```python
from build123d import *

# Parameters (mm, degrees)
SKETCH1_R               = 29.75
BOSS_EXTRUDE1_DEPTH     = 40
CUT_EXTRUDE1_DEPTH      = 4
CUT_EXTRUDE1_DEPTH_BACK = 4
CUT_EXTRUDE1_START      = -20
CUT_EXTRUDE3_START      = -16
CUT_EXTRUDE3_DEPTH      = 16


with BuildPart() as part:
    # Sketch1 → Boss-Extrude1 (new body)
    with BuildSketch(Plane.XY):
        Circle(SKETCH1_R)
        with BuildLine():
            Line((1.5, 2), (1.5, 3.97649343))
            ThreePointArc((1.5, 3.97649343), (0, 4.25), (-1.5, 3.97649343))
            Line((-1.5, 3.97649343), (-1.5, 2))
            ThreePointArc((-1.5, 2), (-2.5, 0), (-1.5, -2))
            Line((-1.5, -2), (-1.5, -3.97649343))
            ThreePointArc((-1.5, -3.97649343), (0, -4.25), (1.5, -3.97649343))
            Line((1.5, -3.97649343), (1.5, -2))
            ThreePointArc((1.5, -2), (2.5, 0), (1.5, 2))
        make_face(mode=Mode.SUBTRACT)
    extrude(amount=BOSS_EXTRUDE1_DEPTH)

    # Sketch2 → Cut-Extrude1 (cut, two sides: drawn at the far end of the back side and taken through both)
    with BuildSketch(Plane.XY.offset(40).offset(CUT_EXTRUDE1_START - CUT_EXTRUDE1_DEPTH_BACK)):
        with BuildLine():
            Line((2.621054601, -11.710255026), (6.498031199, -29.031673919))
            ThreePointArc((6.498031199, -29.031673919), (3.268807192, -29.569873174), (0, -29.75))
            Line((0, -29.75), (0, -12))
            ThreePointArc((0, -12), (1.318510464, -11.927343801), (2.621054601, -11.710255026))
        make_face()
        with BuildLine():
            Line((5.202633875, -10.813537847), (12.898196481, -26.808562579))
            ThreePointArc((12.898196481, -26.808562579), (9.874487797, -28.06344581), (6.731205322, -28.978498493))
            Line((6.731205322, -28.978498493), (2.715108029, -11.688806115))
            ThreePointArc((2.715108029, -11.688806115), (3.982986674, -11.319709234), (5.202633875, -10.813537847))
        make_face()
        with BuildLine():
            Line((7.514375173, -9.355969525), (18.62938845, -23.195007781))
            ThreePointArc((18.62938845, -23.195007781), (15.968021699, -25.101489657), (13.113292322, -26.704008397))
            Line((13.113292322, -26.704008397), (5.289395222, -10.771364732))
            ThreePointArc((5.289395222, -10.771364732), (6.440882702, -10.124970618), (7.514375173, -9.355969525))
        make_face()
        with BuildLine():
            Line((9.436378538, -7.413147786), (23.394355125, -18.378428885))
            ThreePointArc((23.394355125, -18.378428885), (21.233363816, -20.837628489), (18.815249924, -23.044497614))
            Line((18.815249924, -23.044497614), (7.589344507, -9.295259542))
            ThreePointArc((7.589344507, -9.295259542), (8.564718178, -8.405093844), (9.436378538, -7.413147786))
        make_face()
        with BuildLine():
            Line((10.868958019, -5.085838336), (26.945958422, -12.608640875))
            ThreePointArc((26.945958422, -12.608640875), (25.397423769, -15.493010227), (23.541342405, -18.189769041))
            Line((23.541342405, -18.189769041), (9.495667525, -7.337049697))
            ThreePointArc((9.495667525, -7.337049697), (10.244338999, -6.249281436), (10.868958019, -5.085838336))
        make_face()
        with BuildLine():
            Line((11.737811955, -2.494748588), (29.099992138, -6.184897541))
            ThreePointArc((29.099992138, -6.184897541), (28.244229893, -9.344836957), (27.046447919, -12.391616317))
            Line((27.046447919, -12.391616317), (10.909491598, -4.998299019))
            ThreePointArc((10.909491598, -4.998299019), (11.392630545, -3.769345999), (11.737811955, -2.494748588))
        make_face()
        with BuildLine():
            Line((11.997876673, 0.225732911), (29.744735918, 0.559629508))
            ThreePointArc((29.744735918, 0.559629508), (29.626130745, -2.711987667), (29.148771898, -5.95076439))
            Line((29.148771898, -5.95076439), (11.757487825, -2.400308325))
            ThreePointArc((11.757487825, -2.400308325), (11.950035931, -1.093910992), (11.997876673, 0.225732911))
        make_face()
        with BuildLine():
            Line((11.635663748, 2.934506626), (28.846749709, 7.275131011))
            ThreePointArc((28.846749709, 7.275131011), (29.471453141, 4.061520619), (29.739275948, 0.798727786))
            Line((29.739275948, 0.798727786), (11.995674332, 0.322175914))
            ThreePointArc((11.995674332, 0.322175914), (11.887644965, 1.638260418), (11.635663748, 2.934506626))
        make_face()
        with BuildLine():
            Line((10.669959589, 5.491080255), (26.452608147, 13.613303133))
            ThreePointArc((26.452608147, 13.613303133), (27.788219537, 10.624375509), (28.787333194, 7.506793428))
            Line((28.787333194, 7.506793428), (11.611697423, 3.02795029))
            ThreePointArc((11.611697423, 3.02795029), (11.208693595, 4.28546239), (10.669959589, 5.491080255))
        make_face()
        with BuildLine():
            Line((9.150851066, 7.762855451), (22.686484935, 19.245412473))
            ThreePointArc((22.686484935, 19.245412473), (24.663731933, 16.636190283), (26.342316763, 13.825514368))
            Line((26.342316763, 13.825514368), (10.625472308, 5.576678065))
            ThreePointArc((10.625472308, 5.576678065), (9.948396074, 6.710396081), (9.150851066, 7.762855451))
        make_face()
        with BuildLine():
            Line((7.157127728, 9.632005123), (17.743712492, 23.879346034))
            ThreePointArc((17.743712492, 23.879346034), (20.260043902, 21.785158276), (22.531039016, 19.427166053))
            Line((22.531039016, 19.427166053), (9.088150191, 7.83616782))
            ThreePointArc((9.088150191, 7.83616782), (8.172118549, 8.787290733), (7.157127728, 9.632005123))
        make_face()
        with BuildLine():
            Line((4.792195325, 11.001584611), (11.880650911, 27.274761849))
            ThreePointArc((11.880650911, 27.274761849), (14.805555575, 25.804224928), (17.551174341, 24.021215191))
            Line((17.551174341, 24.021215191), (7.07946528, 9.689229657))
            ThreePointArc((7.07946528, 9.689229657), (5.971988803, 10.408426862), (4.792195325, 11.001584611))
        make_face()
        with BuildLine():
            Line((2.178712609, 11.80055979), (5.401391677, 29.25555448))
            ThreePointArc((5.401391677, 29.25555448), (8.583167521, 28.484938745), (11.661006643, 27.369388449))
            Line((11.661006643, 27.369388449), (4.703599318, 11.039753324))
            ThreePointArc((4.703599318, 11.039753324), (3.462117992, 11.489723191), (2.178712609, 11.80055979))
        make_face()
        with BuildLine():
            Line((-0.547770447, 11.987491295), (-1.358014233, 29.718988834))
            ThreePointArc((-1.358014233, 29.718988834), (1.915607925, 29.68826277), (5.166033286, 29.298030652))
            Line((5.166033286, 29.298030652), (2.083778132, 11.817693036))
            ThreePointArc((2.083778132, 11.817693036), (0.772682188, 11.975097588), (-0.547770447, 11.987491295))
        make_face()
    extrude(amount=CUT_EXTRUDE1_DEPTH + CUT_EXTRUDE1_DEPTH_BACK, mode=Mode.SUBTRACT)

    # Sketch3 → Cut-Extrude3 (cut)
    with BuildSketch(Plane.XY.offset(40).offset(CUT_EXTRUDE3_START)):
        with BuildLine():
            Line((0, -12), (0, -18))
            ThreePointArc((0, -18), (1.977765696, -17.891015702), (3.931581902, -17.565382539))
            Line((3.931581902, -17.565382539), (2.621054601, -11.710255026))
            ThreePointArc((2.621054601, -11.710255026), (1.318510464, -11.927343801), (0, -12))
        make_face()
        with BuildLine():
            Line((2.715108029, -11.688806115), (4.072662044, -17.533209172))
            ThreePointArc((4.072662044, -17.533209172), (5.974480012, -16.979563852), (7.803950812, -16.22030677))
            Line((7.803950812, -16.22030677), (5.202633875, -10.813537847))
            ThreePointArc((5.202633875, -10.813537847), (3.982986674, -11.319709234), (2.715108029, -11.688806115))
        make_face()
        with BuildLine():
            Line((5.289395222, -10.771364732), (7.934092833, -16.157047098))
            ThreePointArc((7.934092833, -16.157047098), (9.661324053, -15.187455927), (11.27156276, -14.033954288))
            Line((11.27156276, -14.033954288), (7.514375173, -9.355969525))
            ThreePointArc((7.514375173, -9.355969525), (6.440882702, -10.124970618), (5.289395222, -10.771364732))
        make_face()
        with BuildLine():
            Line((7.589344507, -9.295259542), (11.384016761, -13.942889313))
            ThreePointArc((11.384016761, -13.942889313), (12.847077267, -12.607640767), (14.154567807, -11.119721679))
            Line((14.154567807, -11.119721679), (9.436378538, -7.413147786))
            ThreePointArc((9.436378538, -7.413147786), (8.564718178, -8.405093844), (7.589344507, -9.295259542))
        make_face()
        with BuildLine():
            Line((9.495667525, -7.337049697), (14.243501287, -11.005574546))
            ThreePointArc((14.243501287, -11.005574546), (15.366508499, -9.373922154), (16.303437028, -7.628757504))
            Line((16.303437028, -7.628757504), (10.868958019, -5.085838336))
            ThreePointArc((10.868958019, -5.085838336), (10.244338999, -6.249281436), (9.495667525, -7.337049697))
        make_face()
        with BuildLine():
            Line((10.909491598, -4.998299019), (16.364237396, -7.497448528))
            ThreePointArc((16.364237396, -7.497448528), (17.088945818, -5.654018999), (17.606717932, -3.742122882))
            Line((17.606717932, -3.742122882), (11.737811955, -2.494748588))
            ThreePointArc((11.737811955, -2.494748588), (11.392630545, -3.769345999), (10.909491598, -4.998299019))
        make_face()
        with BuildLine():
            Line((11.757487825, -2.400308325), (17.636231737, -3.600462488))
            ThreePointArc((17.636231737, -3.600462488), (17.925053896, -1.640866488), (17.996815009, 0.338599366))
            Line((17.996815009, 0.338599366), (11.997876673, 0.225732911))
            ThreePointArc((11.997876673, 0.225732911), (11.950035931, -1.093910992), (11.757487825, -2.400308325))
        make_face()
        with BuildLine():
            Line((11.995674332, 0.322175914), (17.993511498, 0.483263871))
            ThreePointArc((17.993511498, 0.483263871), (17.831467447, 2.457390627), (17.453495622, 4.40175994))
            Line((17.453495622, 4.40175994), (11.635663748, 2.934506626))
            ThreePointArc((11.635663748, 2.934506626), (11.887644965, 1.638260418), (11.995674332, 0.322175914))
        make_face()
        with BuildLine():
            Line((11.611697423, 3.02795029), (17.417546134, 4.541925436))
            ThreePointArc((17.417546134, 4.541925436), (16.813040392, 6.428193585), (16.004939383, 8.236620383))
            Line((16.004939383, 8.236620383), (10.669959589, 5.491080255))
            ThreePointArc((10.669959589, 5.491080255), (11.208693595, 4.28546239), (11.611697423, 3.02795029))
        make_face()
        with BuildLine():
            Line((10.625472308, 5.576678065), (15.938208462, 8.365017097))
            ThreePointArc((15.938208462, 8.365017097), (14.922594111, 10.065594121), (13.7262766, 11.644283177))
            Line((13.7262766, 11.644283177), (9.150851066, 7.762855451))
            ThreePointArc((9.150851066, 7.762855451), (9.948396074, 6.710396081), (10.625472308, 5.576678065))
        make_face()
        with BuildLine():
            Line((9.088150191, 7.83616782), (13.632225287, 11.75425173))
            ThreePointArc((13.632225287, 11.75425173), (12.258177823, 13.1809361), (10.735691592, 14.448007684))
            Line((10.735691592, 14.448007684), (7.157127728, 9.632005123))
            ThreePointArc((7.157127728, 9.632005123), (8.172118549, 8.787290733), (9.088150191, 7.83616782))
        make_face()
        with BuildLine():
            Line((7.07946528, 9.689229657), (10.61919792, 14.533844485))
            ThreePointArc((10.61919792, 14.533844485), (8.957983205, 15.612640292), (7.188292988, 16.502376917))
            Line((7.188292988, 16.502376917), (4.792195325, 11.001584611))
            ThreePointArc((4.792195325, 11.001584611), (5.971988803, 10.408426862), (7.07946528, 9.689229657))
        make_face()
        with BuildLine():
            Line((4.703599318, 11.039753324), (7.055398977, 16.559629986))
            ThreePointArc((7.055398977, 16.559629986), (5.193176987, 17.234584787), (3.268068914, 17.700839686))
            Line((3.268068914, 17.700839686), (2.178712609, 11.80055979))
            ThreePointArc((2.178712609, 11.80055979), (3.462117992, 11.489723191), (4.703599318, 11.039753324))
        make_face()
        with BuildLine():
            Line((2.083778132, 11.817693036), (3.125667198, 17.726539554))
            ThreePointArc((3.125667198, 17.726539554), (1.159023282, 17.962646382), (-0.821655671, 17.981236942))
            Line((-0.821655671, 17.981236942), (-0.547770447, 11.987491295))
            ThreePointArc((-0.547770447, 11.987491295), (0.772682188, 11.975097588), (2.083778132, 11.817693036))
        make_face()
    extrude(amount=CUT_EXTRUDE3_DEPTH, mode=Mode.SUBTRACT)


solid = part.part
```
Can you work these out from the model? Positions are in its coordinate system, mm. A direction names the side the tool comes from. Coordinates: 2 decimals unless noted, no trailing zeros. Order: outer loops, then holes, each group sorted by start corner. A loop starts at its lowest first (then second) coordinate and runs counter-clockwise, first axis right, second up. Notation, with made-up numbers: (26, 9.5) - (69, 9.5) arc R33 ccw to (69, 48.5) - close; hole circle Ø5 at (-11, -28.75). An arc over 180 degrees is marked (long way). Answer in a Markdown table with one row per item.
1. Suppose I cut it at B-B (y = -15). Please give me the cut outline in (x, z).
Reply:
| item | result |
|---|---|
| outline | (-25.69, 0) - (25.69, 0) - (25.69, 16) - (19.41, 16) - (19.41, 24) - (25.69, 24) - (25.69, 40) - (9.95, 40) - (9.95, 24) - (12.05, 24) - (12.05, 16) - (7.37, 16) - (7.37, 40) - (7.22, 40) - (7.22, 16) - (3.48, 16) - (3.48, 40) - (3.36, 40) - (3.36, 16) - (0, 16) - (0, 40) - (-25.69, 40) - close; hole (12.25, 16) - (19.09, 16) - (19.09, 24) - (12.25, 24) - close |
2. If I drill on line 1 along Z through (x, y) = (6.5, -23.5); line 2 along Y through (x, z) = (6.5, 36.5); line 3 along X through (y, z) = (2, 11.5), over which ranges is the centre line in solid material (lowest first)?
Reply:
| item | result |
|---|---|
| line 1 | z = 0 to 16, 24 to 40 |
| line 2 | y = -29.03 to -16.79, -13.51 to -13.24, -10.09 to 10.09, 14.92 to 15.26, 16.79 to 29.03 |
| line 3 | x = -29.68 to -1.5, 1.5 to 29.68 |
3. For pin 1 (6 mm diameter, centred on x = 7, z = 24.5, fed in from -Y); pin 2 (4 mm diameter, centred on y = -6.5, z = 6, fed in from -X); pin 3 (2 mm diameter, centred on y = 3, z = 17, fed in from -X), each with a flat end and sliding along its axis, tell me the tip position at first contact or that it passes through.
Reply:
| item | result |
|---|---|
| pin 1 | stops at y = -29.48 |
| pin 2 | stops at x = -29.41 |
| pin 3 | stops at x = -29.68 |
4. For faces 1 (the flat face through (1, 23, 16)), 2 (the flat face through (3, -23, 16)), 3 (the cylindrical face through (15.35, -9.4, 31.89)), 4 (the flat face through (1.5, -3, 20)), 5 (the flat face through (8, -22, 16)), which set-ups out of +Z, -Z, +X, -X, +Y, -Y let a thin tool reach every point of the face, with its end or its side?
Reply:
| item | result |
|---|---|
| face 1 | +Y |
| face 2 | -Y |
| face 3 | +Z |
| face 4 | +Z, -Z |
| face 5 | none |
5. If we mould it in two halves opening along X, with no side actions, what happens to faces 6 (the cylindrical face through (-29.72, 1.31, 19.72)), 7 (the cylindrical face through (-0.02, -4.25, 19.72)), 8 (the flat face through (23, -2, 16))? For each: pulls with the +X half, pulls with the -X half, needs draft (parallel to the pull), parting line crosses it, or undercut.
Reply:
| item | result |
|---|---|
| face 6 | parting line crosses it |
| face 7 | undercut |
| face 8 | needs draft |
6. Suppose I cut it at A-A (z = 5). Please give me the cut outline in (x, y), and give its area (3 significant figures).
Reply:
| item | result |
|---|---|
| outline | circle Ø59.5 at (0, 0); hole (-1.5, -3.98) arc R4.25 ccw to (1.5, -3.98) - (1.5, -2) arc R2.5 ccw to (1.5, 2) - (1.5, 3.98) arc R4.25 ccw to (-1.5, 3.98) - (-1.5, 2) arc R2.5 ccw to (-1.5, -2) - close |
| area | 2,750 mm^2 |
7. Suppose I cut it at C-C (x = -17.5). Please give me the cut outline in (y, z).
Reply:
| item | result |
|---|---|
| outline | (-24.06, 0) - (24.06, 0) - (24.06, 40) - (-24.06, 40) - close |
